Part model, mm, in its own coordinate system. A direction names the side the tool comes from. Round coordinates to 2 decimals unless told otherwise and drop trailing zeros. Write each loop counter-clockwise with the first axis right and the second up, starting at its lowest first coordinate (ties: lowest second). Pieces come first, ordered by that corner, then holes. Notation, with made-up numbers: M -26.5,44 L 1.5,44 A24 cw 1.5,64 Z; hole C 51,2.5 d2. An arc over 180 degrees is marked long. Answer as a JSON object with one key per item and string values. Group by question number.
1. Band-saw the part on C-C, the plane y = 11.5. Write the cut outline in (x, z).
2. Which spindle directions (+Z, -Z, +X, -X, +Y, -Y) get a long thin tool onto all of the face, cutting with end or side? Do faces 4 (the face through (-4, -1, 0)), 5 (the face through (-3.75, -1, 0)), 6 (the face through (5.75, 14.75, 0.08)), 7 (the face through (4, -1, 0)), 8 (the face through (-5.75, 14.75, -0.08)). Say none if no direction does.
3. Two-plate mould, pull along X, no slides. Class faces 1 (the face through (6, 7, 0)), 2 (the face through (0, 19, 5)), 3 (the face through (0, -1, 0)): +X half, -X half, draft (parallel to the pull), parting line (faces both ways), or undercut.
4. Drop flat-ended pins along their axis: pin 1 (1.6 mm diameter, centred on y = -1.5, z = -0.5, fed in from -X); pin 2 (3 mm diameter, centred on y = 9.5, z = 2, fed in from -X); pin 3 (1.5 mm diameter, centred on x = 0.5, z = -0.5, fed in from -Y). Give the stop position or say it passes through.
5. Band-saw the part on B-B, the plane x = 0. Write the cut outline in (y, z).
6. Band-saw the part on D-D, the plane x = -5. Write the cut outline in (y, z).
7. Band-saw the part on A-A, the plane z = 0. Write the cut outline in (x, y), plus the area to 3 significant figures.
8. Drill centre lines: line 1 (Y direction, x = 5, z = 3.25); line 2 (Y direction, x = 3.25, z = -2.75); line 3 (Y direction, x = 5, z = -4.25). Where is each one in solid material? Low to high. Write a range as from..to.
Autodesk Inventor part; units mm, degrees
ref_plane "YZ Plane" through (0, 0, 0) normal (1, 0, 0) x (0, 1, 0)
ref_plane "XZ Plane" through (0, 0, 0) normal (0, 1, 0) x (-1, 0, 0)
ref_plane "XY Plane" through (0, 0, 0) normal (0, 0, 1) x (1, 0, 0)
sketch "スケッチ1" plane through (0, 0, 0) normal (0, 1, 0) x (-1, 0, 0)
  circle A0 centre (0, 0) radius 6
  line L0 (3.3166, 5) -> (-3.3166, 5)
  line L1 (-3.3166, 5) -> (-3.3166, -5)
  line L2 (-3.3166, -5) -> (3.3166, -5)
  line L3 (3.3166, -5) -> (3.3166, 5)
  dimension "d0" = 12
  dimension "d1" = 10
extrude "押し出し1" add sketch "スケッチ1" along normal blind 15 contours A0 L3 | L3 L2 L1 L0 | L1 A0
sketch "スケッチ2" plane through (0, 0, 0) normal (0, -1, 0) x (1, 0, 0)
  circle A0 centre (0, 0) radius 2.5
  dimension "d4" = 5
extrude "押し出し2" add sketch "スケッチ2" along normal blind 1
sketch "スケッチ3" plane through (0, 0, 0) normal (0, -1, 0) x (1, 0, 0)
  line L0 (4, -0.75) -> (-4, -0.75)
  line L1 (-4, -0.75) -> (-4, 0.75)
  line L2 (-4, 0.75) -> (4, 0.75)
  line L3 (4, 0.75) -> (4, -0.75)
  line L4 (3.75, -0.75) -> (-3.75, -0.75)
  line L5 (-3.75, -0.75) -> (-3.75, 0.75)
  line L6 (-3.75, 0.75) -> (3.75, 0.75)
  line L7 (3.75, 0.75) -> (3.75, -0.75)
  point P0 (0, 0)
  point P1 (4, 0)
  point P2 (0, -0.75)
  point P3 (0, 0.75)
  dimension "d7" = 8
  dimension "d8" = 1.5
  dimension "d9" = 7.5
extrude "押し出し3" add sketch "スケッチ3" along normal blind 2 contours L0 L7 L2 L3 | L0 L1 L2 L5
sketch "スケッチ4" plane through (0, 15, 0) normal (0, 1, 0) x (1, 0, 0)
  line L0 (-6, 5) -> (6, 5)
  line L1 (6, 5) -> (6, -5)
  line L2 (6, -5) -> (-6, -5)
  line L3 (-6, -5) -> (-6, 5)
  line L4 (3.3166, 5) -> (-3.3166, 5)
  arc A0 (3.3166, -5) -> (3.3166, 5) centre (0, 0) ccw
  arc A1 (-3.3166, 5) -> (-3.3166, -5) centre (0, 0) ccw
  line L5 (-3.3166, -5) -> (3.3166, -5)
extrude "押し出し4" add sketch "スケッチ4" along normal blind 9
sketch "スケッチ5" plane through (0, 24, 0) normal (0, 1, 0) x (1, 0, 0)
  circle A0 centre (0, 0) radius 1.5
  line L0 (-1.118, 1) -> (1.118, 1)
  dimension "d14" = 3
  dimension "d27" = 1
extrude "押し出し5" add sketch "スケッチ5" along normal blind 10 contours A0 L0 picked at (0.0594, 0.1702)
sketch "スケッチ6" plane through (0, 15, 0) normal (0, -1, 0) x (1, 0, 0)
  arc A0 (6, 0) -> (3.3166, 5) centre (0, 0) ccw
  line L0 (6, 5) -> (6, 0)
  line L1 (3.3166, 5) -> (6, 5)
  arc A1 (3.3166, -5) -> (6, 0) centre (0, 0) ccw
  line L2 (6, -5) -> (3.3166, -5)
  line L3 (6, 0) -> (6, -5)
  arc A2 (-6, 0) -> (-3.3166, -5) centre (0, 0) ccw
  line L4 (-6, -5) -> (-6, 0)
  line L5 (-3.3166, -5) -> (-6, -5)
  arc A3 (-3.3166, 5) -> (-6, 0) centre (0, 0) ccw
  line L6 (-6, 5) -> (-3.3166, 5)
  line L7 (-6, 0) -> (-6, 5)
  arc A4 (1.118, -1) -> (-1.118, -1) centre (0, 0) ccw
  line L8 (-6, -5) -> (-6, 5)
  line L9 (-6, 5) -> (6, 5)
  line L10 (6, 5) -> (6, -5)
  line L11 (6, -5) -> (-6, -5)
  circle A5 centre (0, 0) radius 5.75
  line L12 (3.2404, -4.75) -> (-3.2404, -4.75)
  line L13 (-3.2404, -4.75) -> (-3.2404, 4.75)
  line L14 (-3.2404, 4.75) -> (3.2404, 4.75)
  line L15 (3.2404, 4.75) -> (3.2404, -4.75)
  line L16 (-1.118, -1) -> (1.118, -1)
  point P0 (-3.3166, -5)
  point P1 (3.3166, -5)
  dimension "d17" = 11.5
  dimension "d18" = 9.5
extrude "押し出し6" cut sketch "スケッチ6" along normal blind 0.5 contours A1 L11 A5 L9 A0 | A0 L1 L0 | L3 L2 A1 | A5 L14 L9 | L11 A5 L12 | A5 L11 A2 A3 L9 | A3 L7 L6 | L5 L4 A2
properties part number "motor_6V_60RPM" material "アルミニウム 6061"
Worked answers:
{
 "1": {"outline": "M -3.32,-5 L 3.32,-5 A6 ccw 3.32,5 L -3.32,5 A6 ccw Z"},
 "2": {"face 4": "+Z, -Z, -X, -Y", "face 5": "+Z, -Z, -Y", "face 6": "+X", "face 7": "+Z, -Z, +X, -Y", "face 8": "-X"},
 "3": {"face 1": "+X half", "face 2": "draft", "face 3": "undercut"},
 "4": {"pin 1": "stops at x = -4", "pin 2": "stops at x = -5.98", "pin 3": "stops at y = -1"},
 "5": {"outline": "M -1,-2.5 L 0,-2.5 L 0,-5 L 14.5,-5 L 14.5,-4.75 L 15,-4.75 L 15,-5 L 24,-5 L 24,-1 L 34,-1 L 34,1.5 L 24,1.5 L 24,5 L 15,5 L 15,4.75 L 14.5,4.75 L 14.5,5 L 0,5 L 0,2.5 L -1,2.5 Z"},
 "6": {"outline": "M 0,-3.32 L 14.5,-3.32 L 14.5,-2.84 L 15,-2.84 L 15,-5 L 24,-5 L 24,5 L 15,5 L 15,2.84 L 14.5,2.84 L 14.5,3.32 L 0,3.32 Z"},
 "7": {"outline": "M -6,0 L -4,0 L -4,-2 L -3.75,-2 L -3.75,0 L -2.5,0 L -2.5,-1 L 2.5,-1 L 2.5,0 L 3.75,0 L 3.75,-2 L 4,-2 L 4,0 L 6,0 L 6,14.5 L 5.75,14.5 L 5.75,15 L 6,15 L 6,24 L 1.5,24 L 1.5,34 L -1.5,34 L -1.5,24 L -6,24 L -6,15 L -5.75,15 L -5.75,14.5 L -6,14.5 Z", "area": "324 mm^2"},
 "8": {"line 1": "y = 0..14.5, 15..24", "line 2": "y = 0..24", "line 3": "y = 15..24"}
}
